from build123d import *

# Parameters (mm, degrees)
SKETCH1_W            = 13
SKETCH1_H            = 16
BOSS_EXTRUDE1_DEPTH  = 4
SKETCH2_R            = 1.65
CUT_EXTRUDE1_DEPTH   = 10
SKETCH3_W            = 4
SKETCH3_H            = 13
BOSS_EXTRUDE2_DEPTH  = 4
SKETCH4_W            = 13
SKETCH4_H            = 4
BOSS_EXTRUDE3_DEPTH  = 60
SKETCH6_W            = 4
SKETCH6_H            = 21
SKETCH6_H_2          = 13
BOSS_EXTRUDE4_DEPTH  = 28
SKETCH12_W           = 4
SKETCH12_H           = 28
BOSS_EXTRUDE8_DEPTH  = 1.65
SKETCH13_W           = 4
SKETCH13_H           = 28
BOSS_EXTRUDE9_DEPTH  = 1.65
SKETCH14_W           = 4
SKETCH14_H           = 35.878399396
CUT_EXTRUDE5_DEPTH   = 24
SKETCH15_R           = 1.65
CUT_EXTRUDE6_DEPTH   = 24
SKETCH16_W           = 4
SKETCH16_H           = 11.121600604
SKETCH16_H_2         = 11.3
BOSS_EXTRUDE10_DEPTH = 29.15
SKETCH17_R           = 1.65
CUT_EXTRUDE8_DEPTH   = 29.15
SKETCH18_W           = 22.65
SKETCH18_H           = 4
SKETCH18_W_2         = 13
BOSS_EXTRUDE11_DEPTH = 4
SKETCH19_W           = 4
SKETCH19_H           = 20
BOSS_EXTRUDE12_DEPTH = 40
SKETCH20_R           = 1.65
CUT_EXTRUDE9_DEPTH   = 40


with BuildPart() as part:
    # Sketch1 → Boss-Extrude1 (new body)
    with BuildSketch(Plane(origin=(0, 0, 0), x_dir=(0, 0, -1), z_dir=(1, 0, 0))):
        with Locations((6.5, -8)):
            Rectangle(SKETCH1_W, SKETCH1_H)
    extrude(amount=BOSS_EXTRUDE1_DEPTH)

    # Sketch2 → Cut-Extrude1 (cut)
    with BuildSketch(Plane(origin=(4, 0, 0), x_dir=(0, 0, -1), z_dir=(1, 0, 0))):
        with Locations((6.5, -4)):
            Circle(SKETCH2_R)
        with Locations((6.5, -12)):
            Circle(SKETCH2_R)
    extrude(amount=-CUT_EXTRUDE1_DEPTH, mode=Mode.SUBTRACT)

    # Sketch3 → Boss-Extrude2 (add)
    with BuildSketch(Plane.XZ.offset(16)):
        with Locations((2, -6.5)):
            Rectangle(SKETCH3_W, SKETCH3_H)
    extrude(amount=BOSS_EXTRUDE2_DEPTH)

    # Sketch4 → Boss-Extrude3 (add)
    with BuildSketch(Plane(origin=(4, 0, 0), x_dir=(0, 0, -1), z_dir=(1, 0, 0))):
        with Locations((6.5, -18)):
            Rectangle(SKETCH4_W, SKETCH4_H)
    extrude(amount=BOSS_EXTRUDE3_DEPTH)

    # Sketch6 → Boss-Extrude4 (add)
    with BuildSketch(Plane(origin=(0, -16, 0), x_dir=(1, 0, 0), z_dir=(0, 1, 0))):
        with Locations((62, -10.5)):
            Rectangle(SKETCH6_W, SKETCH6_H)
        with Locations((62, 23.5)):
            Rectangle(SKETCH6_W, SKETCH6_H)
        with Locations((62, 6.5)):
            Rectangle(SKETCH6_W, SKETCH6_H_2)
    extrude(amount=BOSS_EXTRUDE4_DEPTH)

    # Sketch12 → Boss-Extrude8 (add)
    with BuildSketch(Plane(origin=(0, 0, -34), x_dir=(-1, 0, 0), z_dir=(0, 0, -1))):
        with Locations((-62, -2)):
            Rectangle(SKETCH12_W, SKETCH12_H)
    extrude(amount=BOSS_EXTRUDE8_DEPTH)

    # Sketch13 → Boss-Extrude9 (add)
    with BuildSketch(Plane.XY.offset(21)):
        with Locations((62, -2)):
            Rectangle(SKETCH13_W, SKETCH13_H)
    extrude(amount=BOSS_EXTRUDE9_DEPTH)

    # Sketch14 → Cut-Extrude5 (cut)
    with BuildSketch(Plane(origin=(0, 12, 0), x_dir=(1, 0, 0), z_dir=(0, 1, 0))):
        with Locations((62, 6.410800302)):
            Rectangle(SKETCH14_W, SKETCH14_H)
    extrude(amount=-CUT_EXTRUDE5_DEPTH, mode=Mode.SUBTRACT)

    # Sketch15 → Cut-Extrude6 (cut)
    with BuildSketch(Plane(origin=(64, 0, 0), x_dir=(0, 0, -1), z_dir=(1, 0, 0))):
        with Locations((-17, -11.5)):
            Circle(SKETCH15_R)
        with Locations((30, -11.5)):
            Circle(SKETCH15_R)
    extrude(amount=-CUT_EXTRUDE6_DEPTH, mode=Mode.SUBTRACT)

    # Sketch16 → Boss-Extrude10 (add)
    with BuildSketch(Plane(origin=(0, 12, 0), x_dir=(1, 0, 0), z_dir=(0, 1, 0))):
        with Locations((62, -17.089199698)):
            Rectangle(SKETCH16_W, SKETCH16_H)
        with Locations((62, 30)):
            Rectangle(SKETCH16_W, SKETCH16_H_2)
    extrude(amount=BOSS_EXTRUDE10_DEPTH)

    # Sketch17 → Cut-Extrude8 (cut)
    with BuildSketch(Plane(origin=(64, 0, 0), x_dir=(0, 0, -1), z_dir=(1, 0, 0))):
        with Locations((-17, 35.5)):
            Circle(SKETCH17_R)
        with Locations((30, 35.5)):
            Circle(SKETCH17_R)
    extrude(amount=-CUT_EXTRUDE8_DEPTH, mode=Mode.SUBTRACT)

    # Sketch18 → Boss-Extrude11 (add)
    with BuildSketch(Plane(origin=(64, 0, 0), x_dir=(0, 0, -1), z_dir=(1, 0, 0))):
        with Locations((-11.325, -18)):
            Rectangle(SKETCH18_W, SKETCH18_H)
        with Locations((24.325, -18)):
            Rectangle(SKETCH18_W, SKETCH18_H)
        with Locations((6.5, -18)):
            Rectangle(SKETCH18_W_2, SKETCH18_H)
    extrude(amount=-BOSS_EXTRUDE11_DEPTH)

    # Sketch19 → Boss-Extrude12 (add)
    with BuildSketch(Plane(origin=(0, 0, -13), x_dir=(-1, 0, 0), z_dir=(0, 0, -1))):
        with Locations((-2, -10)):
            Rectangle(SKETCH19_W, SKETCH19_H)
    extrude(amount=BOSS_EXTRUDE12_DEPTH)

    # Sketch20 → Cut-Extrude9 (cut)
    with BuildSketch(Plane.ZY):
        with Locations((-46.5, -4)):
            Circle(SKETCH20_R)
        with Locations((-46.5, -12)):
            Circle(SKETCH20_R)
    extrude(amount=-CUT_EXTRUDE9_DEPTH, mode=Mode.SUBTRACT)


solid = part.part
Source: CAD feature listing. Evaluate the final solid. Frame: model axes, mm. A direction names the side the tool comes from. Round coordinates to 2 decimals unless told otherwise and drop trailing zeros. Loops run counter-clockwise (first coordinate to the right, second up) from the corner with the lowest first, then second, coordinate; pieces in that order, holes last. Notation, with made-up numbers: M 20,66.25 L 27,66.25 A16 ccw 27,70.25 Z; hole C 19.5,-39 d9. An arc over 180 degrees is marked long. Answer as CSV lines item,"result".
Q1. Reachability of faces 1 (the face through (2, 0, -26)), 2 (the face through (2.03, -13, -5.19)), 3 (the face through (23, -17, 0)), 4 (the face through (32, -18, -13)), 5 (the face through (62, 15, -24.35)) from +Z, -Z, +X, -X, +Y, -Y: full face, straight path, thin tool, end or side. Return the list, or none.
Verdict:
face 1,"+Z, -Z, -X, +Y"
face 2,"-X"
face 3,"+Z, -X, +Y, -Y"
face 4,"-Z, +Y, -Y"
face 5,"+X, +Y"
Q2. Cut plane B-B (z = -30). Return the cut outline in (x, y).
Verdict:
outline,"M 0,-20 L 4,-20 L 4,0 L 0,0 Z; M 60,-20 L 64,-20 L 64,-13.15 L 60,-13.15 Z; M 60,-9.85 L 64,-9.85 L 64,33.85 L 60,33.85 Z; M 60,37.15 L 64,37.15 L 64,41.15 L 60,41.15 Z"
Q3. Cut plane A-A (y = 1). Return the cut outline in (x, z).
Verdict:
outline,"M 60,-35.65 L 64,-35.65 L 64,-24.35 L 60,-24.35 Z; M 60,11.53 L 64,11.53 L 64,22.65 L 60,22.65 Z"
Q4. Contact query for flat-ended pins moving along their axis: pin 1 (4 mm diameter, centred on y = 35.5, z = -30, fed in from -X); pin 2 (4.5 mm diameter, centred on x = 61.5, y = 14.5, fed in from -Z); pin 3 (3 mm diameter, centred on x = 1.5, z = -33.5, fed in from +Y). Output: stop coordinate, or through.
Verdict:
pin 1,"stops at x = 60"
pin 2,"stops at z = -35.65"
pin 3,"stops at y = 0"
Q5. Cut plane D-D (z = 17). Return the cut outline in (x, y).
Verdict:
outline,"M 60,-20 L 64,-20 L 64,-13.15 L 60,-13.15 Z; M 60,-9.85 L 64,-9.85 L 64,33.85 L 60,33.85 Z; M 60,37.15 L 64,37.15 L 64,41.15 L 60,41.15 Z"
Q6. Pull-direction query (X, two-part tool) for faces 6 (the face through (62, 11, -35.65)), 7 (the face through (4, -10, -26)), 8 (the face through (0, -10, -26)); classes: +X half, -X half, draft (parallel to the pull), parting line (faces both ways), or undercut.
Verdict:
face 6,"draft"
face 7,"undercut"
face 8,"-X half"
Q7. Line query: line 1 along Y through (x, z) = (60.8, 17); line 2 along Y through (x, z) = (2, -46.5); line 3 along Z through (x, y) = (62, -11). Output: solid intervals per line, ascending.
Verdict:
line 1,"y = -20 to -13.15, -9.85 to 33.85, 37.15 to 41.15"
line 2,"y = -20 to -13.65, -10.35 to -5.65, -2.35 to 0"
line 3,"z = -35.65 to -31.57, -28.43 to -24.35, 11.53 to 15.43, 18.57 to 22.65"
Q8. Cut plane C-C (y = 35.5). Return the cut outline in (x, z), plus the area to 3 significant figures.
Verdict:
outline,"M 60,-35.65 L 64,-35.65 L 64,-31.65 L 60,-31.65 Z; M 60,-28.35 L 64,-28.35 L 64,-24.35 L 60,-24.35 Z; M 60,11.53 L 64,11.53 L 64,15.35 L 60,15.35 Z; M 60,18.65 L 64,18.65 L 64,22.65 L 60,22.65 Z"
area,"63.3 mm^2"
